The drawing under review shows one solid part. Ordinate dimensions are in mm from its lowest x, y, z. Coordinates: 2 decimals unless noted, no trailing zeros. Loops run counter-clockwise (first coordinate to the right, second up) from the corner with the lowest first, then second, coordinate; pieces in that order, holes last. Notation, with made-up numbers: M 89,60 L 134,60 A21 cw 134,82 Z; hole C 3.25,-9 d8. An arc over 180 degrees is marked long. Use one line per item in the form item = value.
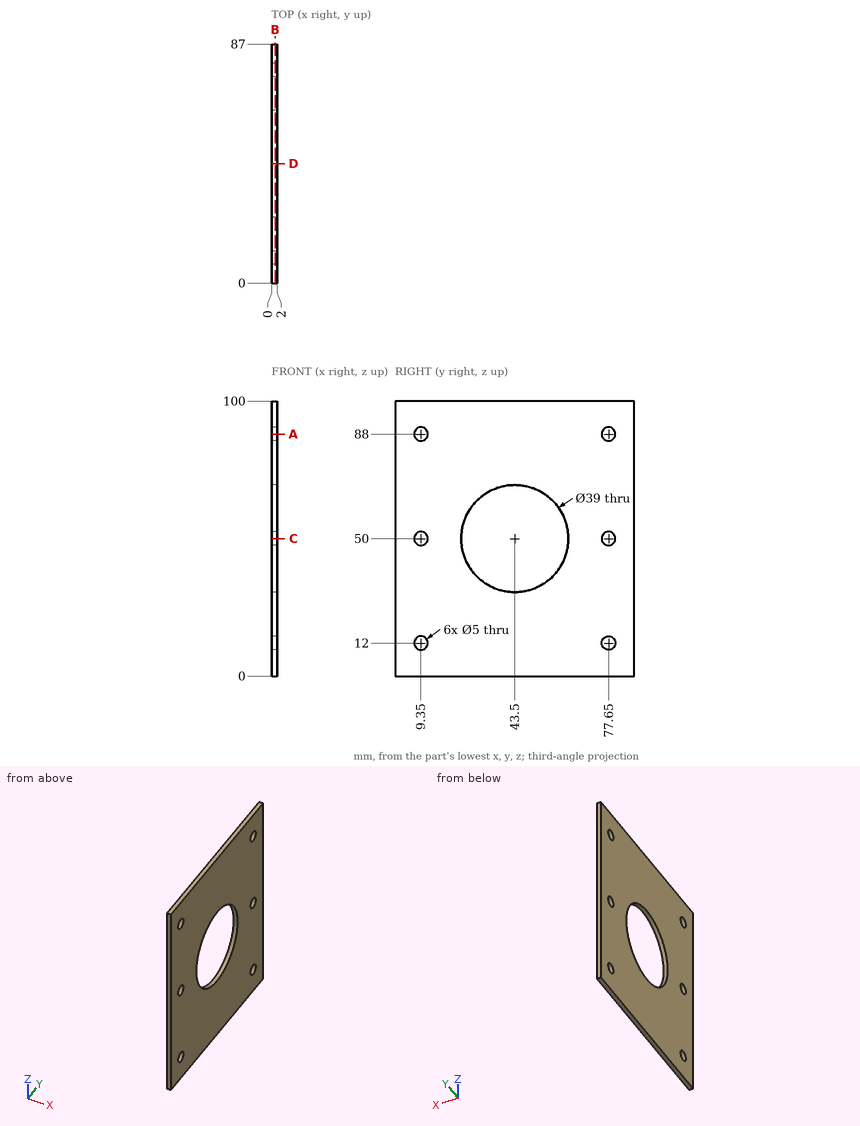
1. Consider section C-C on z = 50. Write out the cut boundary in (x, y), plus the area to 3 significant figures.
Computed values:
outline = M 0,0 L 2,0 L 2,6.85 L 0,6.85 Z; M 0,11.85 L 2,11.85 L 2,24 L 0,24 Z; M 0,63 L 2,63 L 2,75.15 L 0,75.15 Z; M 0,80.15 L 2,80.15 L 2,87 L 0,87 Z
area = 76.0 mm2
2. Consider section D-D on y = 43.5. Write out the cut boundary in (x, z), plus the area to 3 significant figures.
Computed values:
outline = M 0,0 L 2,0 L 2,30.5 L 0,30.5 Z; M 0,69.5 L 2,69.5 L 2,100 L 0,100 Z
area = 122 mm2
3. Consider section B-B on x = 1.25. Write out the cut boundary in (y, z), plus the area to 3 significant figures.
Computed values:
outline = M 0,0 L 87,0 L 87,100 L 0,100 Z; hole C 9.35,12 d5; hole C 9.35,50 d5; hole C 9.35,88 d5; hole C 43.5,50 d39; hole C 77.65,12 d5; hole C 77.65,50 d5; hole C 77.65,88 d5
area = 7,390 mm2
4. Consider section A-A on z = 88. Write out the cut boundary in (x, y), plus the area to 3 significant figures.
Computed values:
outline = M 0,0 L 2,0 L 2,6.85 L 0,6.85 Z; M 0,11.85 L 2,11.85 L 2,75.15 L 0,75.15 Z; M 0,80.15 L 2,80.15 L 2,87 L 0,87 Z
area = 154 mm2
5. Wall thickness on line 1 along Z through (x, y) = (1.3, 9.35); line 2 along Y through (x, z) = (1.6, 13.5); line 3 along Y through (x, z) = (0.8, 48): over which ranges is each line inside the solid? List them lowest first. Write a range as from..to.
Computed values:
line_1 = 0..9.5, 14.5..47.5, 52.5..85.5, 90.5..100
line_2 = 0..7.35, 11.35..75.65, 79.65..87
line_3 = 0..7.85, 10.85..24.1, 62.9..76.15, 79.15..87
6. For pin 1 Ø4.5 at (y, z) = (77.65, 88) entering from +X, flat-tipped, find the tip position at first contact; note if it passes through.
Computed values:
pin_1 = through
